Part print with two shaded views. Sizes in mm from the minimum x, y, z corner. A direction names the side the tool comes from. Coordinates: 2 decimals unless noted, no trailing zeros. Write each loop counter-clockwise with the first axis right and the second up, starting at its lowest first coordinate (ties: lowest second). Pieces come first, ordered by that corner, then holes. Notation, with made-up numbers: (-26, 76.5) - (1, 76.5) arc R17 ccw to (1, 84.5) - close; hole circle Ø2 at (5, -32). An arc over 180 degrees is marked (long way). Answer in a Markdown table with one row per item. Add a question column.
Q1. Band-saw the part on C-C (y = 4). List the corners of the cut face in (x, z) (3 decimals).
Q2. Pin check, flat tips, straight feed: pin 1 (1 mm diameter, centred on x = 13, z = 4, fed in from +Y); pin 2 (6.5 mm diameter, centred on y = 12.5, z = 5, fed in from -X) (3 decimals); pin 3 (4 mm diameter, centred on y = 13, z = 10, fed in from +X) (3 decimals). Stop position of each tip, or through.
Q3. Band-saw the part on B-B (x = 7.62). List the corners of the cut face in (y, z) (1 decimal), and give its area (3 significant figures).
Q4. Band-saw the part on D-D (x = 3.5). List the corners of the cut face in (y, z).
Q5. Drill centre lines: line 1 along X through (y, z) = (14, 7) (3 decimals); line 2 along Y through (x, z) = (5, 7.5); line 3 along Y through (x, z) = (3, 5.5). Where is each one in solid material? Low to high. Write a range as from..to.
Q6. Band-saw the part on A-A (z = 6.35). List the corners of the cut face in (x, y) (1 decimal), and give its area (3 significant figures).
Q7. 3-axis set-ups, long thin cutter, end or side, ignore diameter. For the marked faces 1, 2 and 3: which of +Z, -Z, +X, -X, +Y, -Y reach the whole face in a straight line?
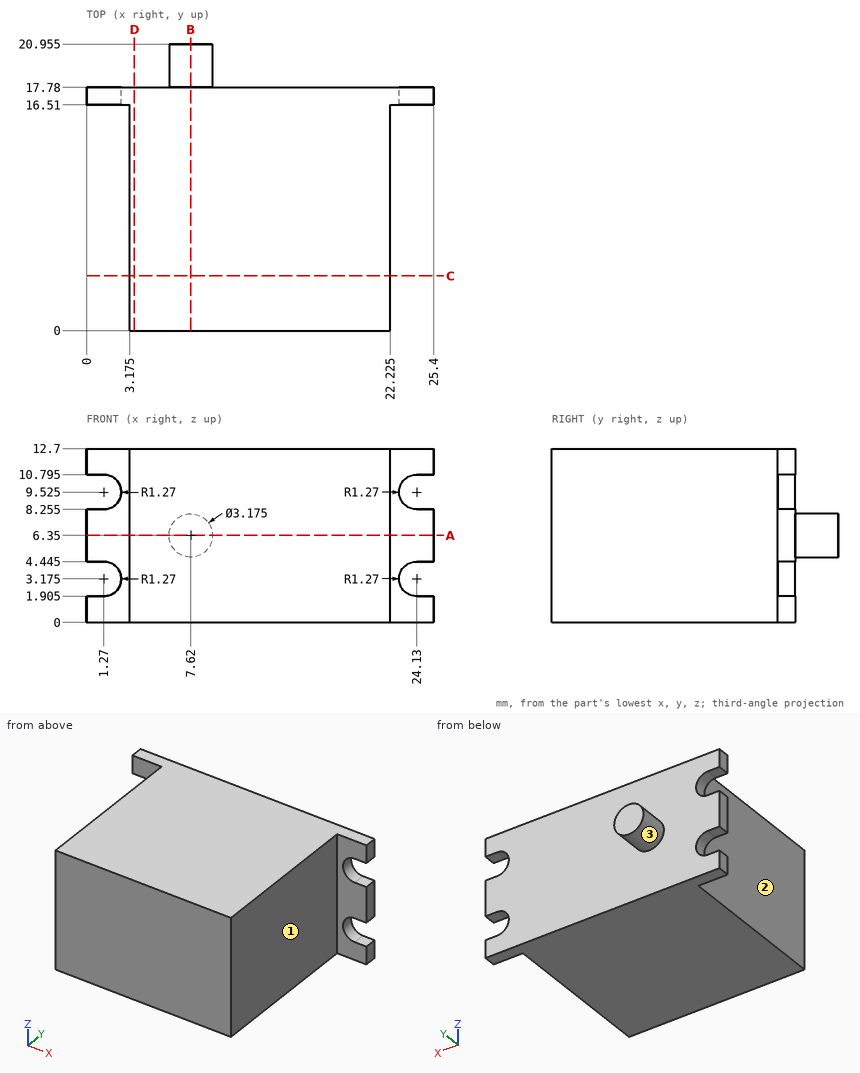
Checked values:
| question | item | result |
|---|---|---|
| 1 | outline | (3.175, 0) - (22.225, 0) - (22.225, 12.7) - (3.175, 12.7) - close |
| 2 | pin 1 | stops at y = 17.78 |
| 2 | pin 2 | stops at x = 3.175 |
| 2 | pin 3 | stops at x = 22.225 |
| 3 | outline | (0, 0) - (17.8, 0) - (17.8, 4.8) - (21, 4.8) - (21, 7.9) - (17.8, 7.9) - (17.8, 12.7) - (0, 12.7) - close |
| 3 | area | 236 mm² |
| 4 | outline | (0, 0) - (17.78, 0) - (17.78, 12.7) - (0, 12.7) - close |
| 5 | line 1 | x = 3.175..22.225 |
| 5 | line 2 | y = 0..17.78 |
| 5 | line 3 | y = 16.51..17.78 |
| 6 | outline | (0, 16.5) - (3.2, 16.5) - (3.2, 0) - (22.2, 0) - (22.2, 16.5) - (25.4, 16.5) - (25.4, 17.8) - (9.2, 17.8) - (9.2, 21) - (6, 21) - (6, 17.8) - (0, 17.8) - close |
| 6 | area | 357 mm² |
| 7 | face 1 | +Z, -Z, +X, -Y |
| 7 | face 2 | +Z, -Z, -X, -Y |
| 7 | face 3 | +Y |
